The listing builds one solid part. Answer for the finished solid, in the listing's coordinates (mm). Face numbers are marked on the shaded views. A direction names the side the tool comes from. Round coordinates to 2 decimals unless told otherwise and drop trailing zeros. Order: outer loops, then holes, each group sorted by start corner. A loop starts at its lowest first (then second) coordinate and runs counter-clockwise, first axis right, second up. Notation, with made-up numbers: M -37.75,-38 L -15.75,-38 A23 cw -15.75,-24 Z; hole C 34.25,-34.5 d6. An arc over 180 degrees is marked long. Write item = value, one per line. Start each with the question number.
(1) For a pull along Z with two mould halves and no side action, classify the marked faces 3, 4 and 5 as released by +Z, released by -Z, zero draft, split by the parting line, or undercut.
(2) A cutting plane is placed at D-D, the plane x = 12.5. Determine the outline of the cut face in (y, z).
(3) A cutting plane is placed at A-A, the plane y = 12. Determine the outline of the cut face in (x, z), and give its area (3 significant figures).
(4) Straight lines are drawn through the part: probe 1 along X at (y, z) = (15, -70); probe 2 along X at (y, z) = (31, -22); probe 3 along Y at (x, z) = (-6.5, -59.5). For each, find the intervals that lie inside material, in ascending order. Write a range as from..to.
(5) A cutting plane is placed at B-B, the plane y = 45. Determine the outline of the cut face in (x, z).
(6) Each of these flat-tipped pins is pushed along its axis until it touches: pin 1 (1.2 mm diameter, centred on x = 10.5, y = 1.5, fed in from -Z); pin 2 (2 mm diameter, centred on x = -8.5, y = 2, fed in from +Z); pin 3 (6.5 mm diameter, centred on x = 68.5, y = 16, fed in from +Z); pin 4 (8 mm diameter, centred on x = 0, z = -41, fed in from -Y). Where does it stop, or does it pass through?
(7) A cutting plane is placed at C-C, the plane z = 17. Determine the outline of the cut face in (x, y).
(8) Which of the six approach directions +Z, -Z, +X, -X, +Y, -Y give full straight-line access (tool end or side, diameter ignored) to the marked faces 1 and 2?
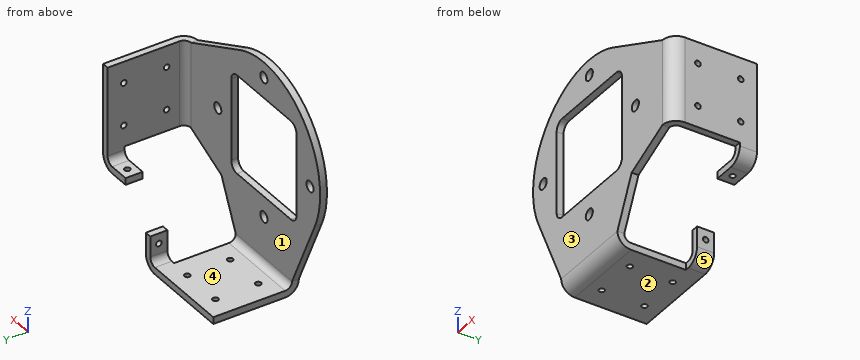
from build123d import *

# Parameters (mm, degrees)
SKETCH_1_R                         = 3.15
EXTRUDE_1_DEPTH                    = 4
SM_EDGE_FLANGE_1_DEPTH             = 50
SM_EDGE_FLANGE_1_BEND_DEPTH        = 50
SKETCH_25_W                        = 10
SKETCH_25_H                        = 10
EXTRUDE_3_DEPTH                    = 4
SKETCH_23_W                        = 10
SKETCH_23_H                        = 10
EXTRUDE_2_DEPTH                    = 4
SKETCH_21_R                        = 1.65
CUT_EXTRUDE_1_DEPTH                = 149.290255917
SKETCH_22_R                        = 1.65
CUT_EXTRUDE_2_DEPTH                = 149.290255917
SM_EDGE_FLANGE_2_STRIP_W           = 24
SM_EDGE_FLANGE_2_STRIP_H           = 4
SM_EDGE_FLANGE_2_STRIP_CUT_DEPTH   = 10
SM_EDGE_FLANGE_2_STRIP_2_W         = 24
SM_EDGE_FLANGE_2_STRIP_2_H         = 4
SM_EDGE_FLANGE_2_STRIP_CUT_2_DEPTH = 10
SM_EDGE_FLANGE_2_DEPTH             = 10
SM_EDGE_FLANGE_2_BEND_DEPTH        = 10
SKETCH_38_R                        = 1.65
CUT_EXTRUDE_3_DEPTH                = 4
SKETCH_37_R                        = 1.65
CUT_EXTRUDE_4_DEPTH                = 4


# Sheet-metal steps are written as plain solids
with BuildPart() as part:
    # Sketch 1 → 凸台-拉伸1 (new body)
    with BuildSketch(Plane(origin=(0, 0, 0), x_dir=(1, 0, 0), z_dir=(0, 1, 0))):
        with BuildLine():
            Line((-25, 65), (-45.371050591, 21.011134388))
            ThreePointArc((-45.371050591, 21.011134388), (-35.355339059, -35.355339059), (21.011134388, -45.371050591))
            Line((21.011134388, -45.371050591), (65, -25))
            Line((65, -25), (65, 25))
            Line((65, 25), (37.660706721, 37.660706721))
            Line((37.660706721, 37.660706721), (25, 65))
            Line((25, 65), (-25, 65))
        make_face()
        with Locations(Location((0, 41, 0), (0, 0, 270))):
            Circle(SKETCH_1_R, mode=Mode.SUBTRACT)
        with Locations(Location((0, -41, 0), (0, 0, 270))):
            Circle(SKETCH_1_R, mode=Mode.SUBTRACT)
        with Locations(Location((-41, 0, 0), (0, 0, 270))):
            Circle(SKETCH_1_R, mode=Mode.SUBTRACT)
        with BuildLine():
            ThreePointArc((29, -24), (27.535533906, -27.535533906), (24, -29))
            Line((24, -29), (-24, -29))
            ThreePointArc((-24, -29), (-27.535533906, -27.535533906), (-29, -24))
            Line((-29, -24), (-29, 24))
            ThreePointArc((-29, 24), (-27.535533906, 27.535533906), (-24, 29))
            Line((-24, 29), (24, 29))
            ThreePointArc((24, 29), (27.535533906, 27.535533906), (29, 24))
            Line((29, 24), (29, -24))
        make_face(mode=Mode.SUBTRACT)
        with Locations(Location((41, 0, 0), (0, 0, 270))):
            Circle(SKETCH_1_R, mode=Mode.SUBTRACT)
    extrude(amount=EXTRUDE_1_DEPTH)

    # 边线-法兰1 section (across the edge) → 边线-法兰1 (add)
    with BuildSketch(Plane(origin=(69, 4, 25), x_dir=(-1, 0, 0), z_dir=(0, 0, -1))):
        with BuildLine():
            Line((-4, 4), (-4, 46))
            Line((-4, 46), (0, 46))
            Line((0, 46), (0, 4))
            ThreePointArc((0, 4), (1.171572875, 1.171572875), (4, 0))
            Line((4, 0), (4, -4))
            ThreePointArc((4, -4), (-1.656854249, -1.656854249), (-4, 4))
        make_face()
    extrude(amount=SM_EDGE_FLANGE_1_DEPTH)

    # 边线-法兰1 section 2 (across the edge) → 边线-法兰1 bend (add)
    with BuildSketch(Plane(origin=(25, 4, -69), x_dir=(0, 0, 1), z_dir=(-1, 0, 0))):
        with BuildLine():
            Line((-4, 4), (-4, 46))
            Line((-4, 46), (0, 46))
            Line((0, 46), (0, 4))
            ThreePointArc((0, 4), (1.171572875, 1.171572875), (4, 0))
            Line((4, 0), (4, -4))
            ThreePointArc((4, -4), (-1.656854249, -1.656854249), (-4, 4))
        make_face()
    extrude(amount=SM_EDGE_FLANGE_1_BEND_DEPTH)

    # 草图25 → 凸台-拉伸3 (add)
    with BuildSketch(Plane.XY.offset(-69)):
        with Locations((30, 45)):
            Rectangle(SKETCH_25_W, SKETCH_25_H)
    extrude(amount=-EXTRUDE_3_DEPTH)

    # 草图23 → 凸台-拉伸2 (add)
    with BuildSketch(Plane.ZY.offset(-69)):
        with Locations((-30, 45)):
            Rectangle(SKETCH_23_W, SKETCH_23_H)
    extrude(amount=-EXTRUDE_2_DEPTH)

    # 草图21 → 切除-拉伸1 (cut, through all)
    with BuildSketch(Plane.XY.offset(-69)):
        with Locations((-12.5, 40.5)):
            Circle(SKETCH_21_R)
        with Locations(Location((12.5, 40.5, 0), (0, 0, 180))):
            Circle(SKETCH_21_R)
        with Locations((12.5, 15.5)):
            Circle(SKETCH_21_R)
        with Locations(Location((-12.5, 15.5, 0), (0, 0, 180))):
            Circle(SKETCH_21_R)
    extrude(amount=-CUT_EXTRUDE_1_DEPTH, mode=Mode.SUBTRACT)

    # 草图22 → 切除-拉伸2 (cut, through all)
    with BuildSketch(Plane.ZY.offset(-69)):
        with Locations(Location((-12.5, 40.5, 0), (0, 0, 270))):
            Circle(SKETCH_22_R)
        with Locations(Location((12.5, 40.5, 0), (0, 0, 90))):
            Circle(SKETCH_22_R)
        with Locations(Location((12.5, 15.5, 0), (0, 0, 270))):
            Circle(SKETCH_22_R)
        with Locations(Location((-12.5, 15.5, 0), (0, 0, 90))):
            Circle(SKETCH_22_R)
    extrude(amount=-CUT_EXTRUDE_2_DEPTH, mode=Mode.SUBTRACT)

    # 边线-法兰2 strip (across the edge) → 边线-法兰2 strip cut (cut)
    with BuildSketch(Plane(origin=(69, 50, -35), x_dir=(0, 0, 1), z_dir=(0, -1, 0))):
        with Locations((-4, -2)):
            Rectangle(SM_EDGE_FLANGE_2_STRIP_W, SM_EDGE_FLANGE_2_STRIP_H)
    extrude(amount=SM_EDGE_FLANGE_2_STRIP_CUT_DEPTH, mode=Mode.SUBTRACT)

    # 边线-法兰2 strip 2 (across the edge) → 边线-法兰2 strip cut 2 (cut)
    with BuildSketch(Plane(origin=(35, 40, -69), x_dir=(-1, 0, 0), z_dir=(0, 1, 0))):
        with Locations((-4, -2)):
            Rectangle(SM_EDGE_FLANGE_2_STRIP_2_W, SM_EDGE_FLANGE_2_STRIP_2_H)
    extrude(amount=SM_EDGE_FLANGE_2_STRIP_CUT_2_DEPTH, mode=Mode.SUBTRACT)

    # 边线-法兰2 section (across the edge) → 边线-法兰2 (add)
    with BuildSketch(Plane(origin=(69, 50, -35), x_dir=(0, 0, 1), z_dir=(0, -1, 0))):
        with BuildLine():
            Line((0, 4), (0, 16))
            Line((0, 16), (4, 16))
            Line((4, 16), (4, 4))
            ThreePointArc((4, 4), (5.171572875, 1.171572875), (8, 0))
            Line((8, 0), (8, -4))
            ThreePointArc((8, -4), (2.343145751, -1.656854249), (0, 4))
        make_face()
    extrude(amount=SM_EDGE_FLANGE_2_DEPTH)

    # 边线-法兰2 section 2 (across the edge) → 边线-法兰2 bend (add)
    with BuildSketch(Plane(origin=(35, 40, -69), x_dir=(-1, 0, 0), z_dir=(0, 1, 0))):
        with BuildLine():
            Line((0, 4), (0, 16))
            Line((0, 16), (4, 16))
            Line((4, 16), (4, 4))
            ThreePointArc((4, 4), (5.171572875, 1.171572875), (8, 0))
            Line((8, 0), (8, -4))
            ThreePointArc((8, -4), (2.343145751, -1.656854249), (0, 4))
        make_face()
    extrude(amount=SM_EDGE_FLANGE_2_BEND_DEPTH)

    # 草图38 → 切除-拉伸3 (cut)
    with BuildSketch(Plane(origin=(0, 0, -35), x_dir=(-1, 0, 0), z_dir=(0, 0, -1))):
        with Locations((-59, 45)):
            Circle(SKETCH_38_R)
    extrude(amount=-CUT_EXTRUDE_3_DEPTH, mode=Mode.SUBTRACT)

    # 草图37 → 切除-拉伸4 (cut)
    with BuildSketch(Plane(origin=(35, 0, 0), x_dir=(0, 0, -1), z_dir=(1, 0, 0))):
        with Locations((59, 45)):
            Circle(SKETCH_37_R)
    extrude(amount=-CUT_EXTRUDE_4_DEPTH, mode=Mode.SUBTRACT)


solid = part.part
Reported:
q1.face_3 = zero draft
q1.face_4 = released by +Z
q1.face_5 = released by -Z
q2.outline = M 0,-65 A8 ccw 8,-73 L 13.85,-73 L 13.85,-69 L 8,-69 A4 cw 4,-65 L 4,-29 L 0,-29 Z; M 0,29 L 4,29 L 4,48.41 L 0,48.41 Z; M 17.15,-73 L 38.85,-73 L 38.85,-69 L 17.15,-69 Z; M 42.15,-73 L 50,-73 L 50,-69 L 42.15,-69 Z
q3.outline = M -25,-73 L 25,-73 L 25,-69 L -25,-69 Z; M 69,-25 L 73,-25 L 73,25 L 69,25 Z
q3.area = 400 mm²
q4.probe_1 = -25..-14.07, -10.93..10.93, 14.07..25
q4.probe_2 = 69..73
q4.probe_3 = 0..4
q5.outline = M -25,-73 L 27,-73 A8 ccw 35,-65 L 35,-60.65 L 31,-60.65 L 31,-65 A4 cw 27,-69 L -25,-69 Z; M 31,-57.35 L 35,-57.35 L 35,-53 L 31,-53 Z; M 53,-35 L 57.35,-35 L 57.35,-31 L 53,-31 Z; M 60.65,-35 L 65,-35 A8 ccw 73,-27 L 73,25 L 69,25 L 69,-27 A4 cw 65,-31 L 60.65,-31 Z
q6.pin_1 = -70.4
q6.pin_2 = 49.43
q6.pin_3 = 25
q6.pin_4 = 0
q7.outline = M -47.02,0 L -29,0 L -29,4 L -47.02,4 Z; M 29,0 L 65,0 A8 ccw 73,8 L 73,50 L 69,50 L 69,8 A4 cw 65,4 L 29,4 Z
q8.face_1 = +Z, -X, +Y
q8.face_2 = -Z, +X, -X, +Y, -Y
